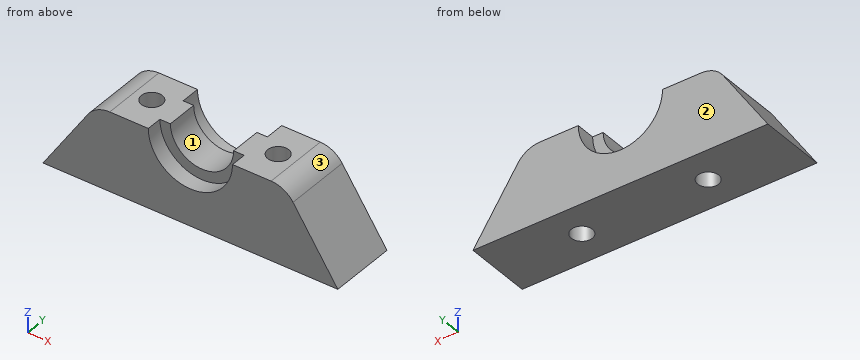
Autodesk Fusion 360 part; units mm, degrees
sketch "Sketch1" plane through (0, 0, 0) normal (0, 1, 0) x (1, 0, 0)
  line L0 (-18, 0) -> (-28, 15)
  line L1 (-28, 15) -> (28, 15)
  line L2 (28, 15) -> (18, 0)
  line L3 (18, 0) -> (-18, 0)
  dimension "d1" = 10
  dimension "d2" = 10
  dimension "d3" = 56
  dimension "d21" = 15
extrude "Extrude1" add sketch "Sketch1" along normal blind 12.7
sketch "Sketch2" plane through (0, 12.7, 0) normal (0, 1, 0) x (-1, 0, 0)
  line L0 (-18, 0) -> (-28, -15)
  line L1 (-28, -15) -> (28, -15)
  line L2 (28, -15) -> (18, 0)
  line L3 (18, 0) -> (-18, 0)
  circle A0 centre (0, 0) radius 8
  circle A1 centre (0, 0) radius 6
  dimension "d7" = 16
  dimension "d8" = 12
extrude "Extrude2" cut sketch "Sketch2" against normal through all contours L3 A1 picked at (-1.4661, -1.3603)
extrude "Extrude3" cut sketch "Sketch2" against normal blind 3.7 contours L3 A0 A1 picked at (7.2812, -0.6955)
extrude "Extrude4" cut sketch "Sketch2" along normal blind 3 from surface at -12.7 contours L3 A0 A1 picked at (7.2812, -0.6955)
sketch "Sketch3" plane through (0, 0, 0) normal (0, 0, 1) x (1, 0, 0)
  line L0 (-8, 3) -> (-6, 3)
  line L1 (-6, 3) -> (-6, 9)
  line L2 (-6, 9) -> (-8, 9)
  line L3 (-8, 9) -> (-8, 12.7)
  line L4 (-8, 12.7) -> (-18, 12.7)
  line L5 (-18, 12.7) -> (-18, 0)
  line L6 (-18, 0) -> (-8, 0)
  line L7 (-8, 0) -> (-8, 3)
  line L8 (-12, 6.35) -> (12, 6.35)
  circle A0 centre (-12, 6.35) radius 2
  circle A1 centre (12, 6.35) radius 2
  dimension "d15" = 24
  dimension "d16" = 12
  dimension "d17" = 6.35
  dimension "d18" = 4
  dimension "d19" = 4
extrude "Extrude5" cut sketch "Sketch3" against normal through all contours A0 | A1
fillet "Fillet1" radius 5 2 edges at (-18, 6.35, 0) (18, 6.35, 0)
equation "d17 = ( 12.7 / 2 ) * 1 mm"
Design review of the part built by this model. Coordinates are the model's own, in mm. Face numbers are marked on the shaded views. Coordinates: 2 decimals unless noted, no trailing zeros. Loops run counter-clockwise (first coordinate to the right, second up) from the corner with the lowest first, then second, coordinate; pieces in that order, holes last. Notation, with made-up numbers: (61.5, 34.5) -> (79.5, 34.5) arc R11 cw to (79.5, 38.5) -> close; hole circle Ø3 at (32, 26). An arc over 180 degrees is marked (long way). Answer as a JSON object with one key per item and string values.
Q1. Take a section at D-D on x = 0. Give the boundary of the cut face in (y, z).
Answer block:
{"outline": "(0, -15) -> (12.7, -15) -> (12.7, -8) -> (9, -8) -> (9, -6) -> (3, -6) -> (3, -8) -> (0, -8) -> close"}
Q2. To check wall thickness, follow L1, parallel to Y at x = -12, z = -4.5; L2, parallel to X at y = 7.25, z = -2.5; L3, parallel to X at y = 5.75, z = -4.5. State the ranges of each line that lie inside material, in increasing order.
Answer block:
{"L1": "y = 0 to 4.35, 8.35 to 12.7", "L2": "x = -19.67 to -13.79, -10.21 to -5.45, 5.45 to 10.21, 13.79 to 19.67", "L3": "x = -21 to -13.91, -10.09 to -3.97, 3.97 to 10.09, 13.91 to 21"}
Q3. The part is to be moulded in two halves that separate along X. For the marked faces 1, 2 and 3, say which applies: +X half, -X half, draft (parallel to the pull), parting line (faces both ways), or undercut.
Answer block:
{"face 1": "undercut", "face 2": "draft", "face 3": "+X half"}
Q4. Take a section at C-C on y = 9.75. Give the boundary of the cut face in (x, z).
Answer block:
{"outline": "(-28, -15) -> (28, -15) -> (19.48, -2.23) arc R5 ccw to (15.32, 0) -> (8, 0) arc R8 cw to (-8, 0) -> (-15.32, 0) arc R5 ccw to (-19.48, -2.23) -> close"}
Q5. Take a section at B-B on y = 6.35. Give the boundary of the cut face in (x, z).
Answer block:
{"outline": "(-28, -15) -> (-14, -15) -> (-14, 0) -> (-15.32, 0) arc R5 ccw to (-19.48, -2.23) -> close; (-10, -15) -> (10, -15) -> (10, 0) -> (6, 0) arc R6 cw to (-6, 0) -> (-10, 0) -> close; (14, -15) -> (28, -15) -> (19.48, -2.23) arc R5 ccw to (15.32, 0) -> (14, 0) -> close"}
Q6. Clearance check with flat-ended pins moving along their axes: pin 1 Ø3 at (y, z) = (10, -9.5) entering from +X; pin 2 Ø6 at (y, z) = (2, -3.5) entering from -X; pin 3 Ø2 at (x, y) = (19.5, 3.5) entering from +Z. State where each tip first meets the part, or that it passes through.
Answer block:
{"pin 1": "stops at x = 25.33", "pin 2": "stops at x = -22.33", "pin 3": "stops at z = -1.14"}
Q7. Take a section at A-A on x = -12. Give the boundary of the cut face in (y, z), plus the area to 4 significant figures.
Answer block:
{"outline": "(0, -15) -> (4.35, -15) -> (4.35, 0) -> (0, 0) -> close; (8.35, -15) -> (12.7, -15) -> (12.7, 0) -> (8.35, 0) -> close", "area": "130.5 mm^2"}
